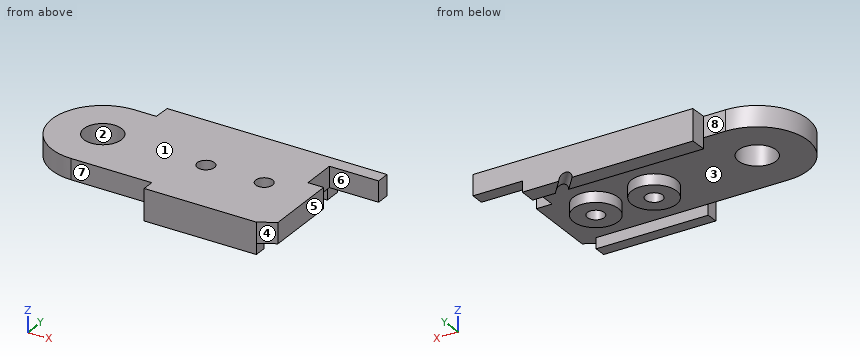
from build123d import *

# Parameters (mm, degrees)
BOSS_EXTRUDE1_DEPTH  = 2
BOSS_EXTRUDE6_DEPTH  = 2.5
CUT_EXTRUDE6_DEPTH   = 2.5
BOSS_EXTRUDE14_DEPTH = 2.3
SKETCH32_R           = 2.1
CUT_EXTRUDE7_DEPTH   = 2.3
SKETCH33_W           = 12.5
SKETCH33_H           = 1.343145751
BOSS_EXTRUDE15_DEPTH = 1.2
SKETCH35_W           = 5.479645997
SKETCH35_H           = 3.827993755
CUT_EXTRUDE8_DEPTH   = 2.4
SKETCH36_W           = 3.7
SKETCH36_H           = 1.827993755
CUT_EXTRUDE9_DEPTH   = 2.4
SKETCH37_R           = 3.9
BOSS_EXTRUDE16_DEPTH = 2.3
CUT_EXTRUDE10_DEPTH  = 5.3
SKETCH43_R           = 2.5
BOSS_EXTRUDE17_DEPTH = 1.2
SKETCH44_R           = 0.95
CUT_EXTRUDE11_DEPTH  = 9
SKETCH45_R           = 2
CUT_EXTRUDE12_DEPTH  = 2.5
SKETCH52_R           = 0.75
CUT_EXTRUDE13_DEPTH  = 10


with BuildPart() as part:
    # Sketch3 → Boss-Extrude1 (new body)
    with BuildSketch(Plane.XY):
        with BuildLine():
            Line((8, 0), (9, -2.5))
            Line((9, -2.5), (9, -7))
            Line((9, -7), (21.5, -7))
            Line((21.5, -7), (25.050252532, -4.949747468))
            ThreePointArc((25.050252532, -4.949747468), (36.467156728, -2.678784027), (30, 7))
            Line((30, 7), (27, 7.5))
            Line((27, 7.5), (5.656854249, 7.5))
            Line((5.656854249, 7.5), (5.656854249, 5.656854249))
            ThreePointArc((5.656854249, 5.656854249), (7.39103626, 3.061467459), (8, 0))
        make_face()
    extrude(amount=BOSS_EXTRUDE1_DEPTH)

    # Sketch22 → Boss-Extrude6 (add)
    with BuildSketch(Plane.XY.offset(2)):
        with BuildLine():
            Line((5.656854249, 5.656854249), (2.486790148, 5.656854249))
            Line((2.486790148, 5.656854249), (2.486790148, 7.5))
            Line((2.486790148, 7.5), (5.656854249, 7.5))
            Line((5.656854249, 7.5), (21.5, 7.5))
            Line((21.5, 7.5), (27, 7.5))
            Line((27, 7.5), (27, 2.172006245))
            Line((27, 2.172006245), (23.275126266, 2.172006245))
            Line((23.275126266, 2.172006245), (23.275126266, -5.974873734))
            Line((23.275126266, -5.974873734), (21.5, -7))
            Line((21.5, -7), (9, -7))
            Line((9, -7), (9, -2.5))
            Line((9, -2.5), (8, 0))
            ThreePointArc((8, 0), (7.39103626, 3.061467459), (5.656854249, 5.656854249))
        make_face()
    extrude(amount=BOSS_EXTRUDE6_DEPTH)

    # Sketch26 → Cut-Extrude6 (cut)
    with BuildSketch(Plane.XY.offset(2)):
        Polygon((18.098080448, 5.3), (2.530052458, 5.3), (2.530052458, 4), (18.098080448, 4), (27, 4), (27, 5.3), align=None)
    extrude(amount=CUT_EXTRUDE6_DEPTH, mode=Mode.SUBTRACT)


with BuildPart() as body_2:
    # Sketch31 → Boss-Extrude14 (new body)
    with BuildSketch(Plane.XY.offset(4.5)):
        with BuildLine():
            Line((2.432688066, 5.656854249), (0, 5.656854249))
            ThreePointArc((0, 5.656854249), (-5.656854249, 0), (0, -5.656854249))
            Line((0, -5.656854249), (9, -5.656854249))
            Line((9, -5.656854249), (9, -7))
            Line((9, -7), (21.5, -7))
            Line((21.5, -7), (23.275126266, -5.974873734))
            Line((23.275126266, -5.974873734), (23.275126266, 2.172006245))
            Line((23.275126266, 2.172006245), (27, 2.172006245))
            Line((27, 2.172006245), (27, 7.5))
            Line((27, 7.5), (2.486790148, 7.5))
            Line((2.486790148, 7.5), (2.432688066, 5.656854249))
        make_face()
    extrude(amount=BOSS_EXTRUDE14_DEPTH)

    # Sketch32 → Cut-Extrude7 (cut)
    with BuildSketch(Plane.XY.offset(6.8)):
        Circle(SKETCH32_R)
    extrude(amount=-CUT_EXTRUDE7_DEPTH, mode=Mode.SUBTRACT)

    # Sketch33 → Boss-Extrude15 (add)
    with BuildSketch(Plane.XY.offset(6.8)):
        with Locations((15.25, -6.328427125)):
            Rectangle(SKETCH33_W, SKETCH33_H)
        Polygon((2.486790148, 7.5), (21.5, 7.5), (21.5, 5.656854249), (2.432688066, 5.656854249), align=None)
    extrude(amount=BOSS_EXTRUDE15_DEPTH)


with BuildPart() as cut_extrude8_tool:
    # Sketch35 → Cut-Extrude8 (new body)
    with BuildSketch(Plane.XY.offset(6.8)):
        with Locations((24.260177002, 4.086003123)):
            Rectangle(SKETCH35_W, SKETCH35_H)
    extrude(amount=-CUT_EXTRUDE8_DEPTH)


with BuildPart() as part_1:
    add(part.part)

    # Cut-Extrude8: cut by cut_extrude8_tool
    add(cut_extrude8_tool.part, mode=Mode.SUBTRACT)

    # Sketch36 → Cut-Extrude9 (cut)
    with BuildSketch(Plane.XY.offset(4.4)):
        with Locations((25.15, 3.086003123)):
            Rectangle(SKETCH36_W, SKETCH36_H)
    extrude(amount=-CUT_EXTRUDE9_DEPTH, mode=Mode.SUBTRACT)

    # Sketch37 → Boss-Extrude16 (add)
    with BuildSketch(Plane.XY.offset(2)):
        with Locations((30, 0)):
            Circle(SKETCH37_R)
    extrude(amount=BOSS_EXTRUDE16_DEPTH)

    # Sketch39 → Cut-Extrude10 (cut, through all)
    with BuildSketch(Plane.XY.offset(4.3)):
        with BuildLine():
            Line((29, 1.732050808), (29, -1.732050808))
            ThreePointArc((29, -1.732050808), (32, 0), (29, 1.732050808))
        make_face()
    extrude(amount=-CUT_EXTRUDE10_DEPTH, mode=Mode.SUBTRACT)


with BuildPart() as body_2_1:
    add(body_2.part)

    # Cut-Extrude8: cut by cut_extrude8_tool
    add(cut_extrude8_tool.part, mode=Mode.SUBTRACT)

    # Sketch43 → Boss-Extrude17 (add)
    with BuildSketch(Plane.XY.offset(6.8)):
        with Locations((11.5, 0)):
            Circle(SKETCH43_R)
        with Locations((18, 0)):
            Circle(SKETCH43_R)
    extrude(amount=BOSS_EXTRUDE17_DEPTH)


with BuildPart() as cut_extrude11_tool:
    # Sketch44 → Cut-Extrude11 (new body, through all)
    with BuildSketch(Plane.XY.offset(8)):
        with Locations((11.5, 0)):
            Circle(SKETCH44_R)
        with Locations((18, 0)):
            Circle(SKETCH44_R)
    extrude(amount=-CUT_EXTRUDE11_DEPTH)


with BuildPart() as part_2:
    add(part_1.part)

    # Cut-Extrude11: cut by cut_extrude11_tool
    add(cut_extrude11_tool.part, mode=Mode.SUBTRACT)

    # Sketch45 → Cut-Extrude12 (cut)
    with BuildSketch(Plane(origin=(0, 0, 0), x_dir=(-1, 0, 0), z_dir=(0, 0, -1))):
        with Locations((-11.5, 0)):
            Circle(SKETCH45_R)
        with Locations((-18, 0)):
            Circle(SKETCH45_R)
    extrude(amount=-CUT_EXTRUDE12_DEPTH, mode=Mode.SUBTRACT)


with BuildPart() as body_2_2:
    add(body_2_1.part)

    # Cut-Extrude11: cut by cut_extrude11_tool
    add(cut_extrude11_tool.part, mode=Mode.SUBTRACT)

    # Sketch52 → Cut-Extrude13 (cut, along a direction that is not the sketch's normal)
    with BuildSketch(Plane.XZ.offset(-5.656854249)):
        with Locations((18.235476819, 8)):
            Circle(SKETCH52_R)
    extrude(amount=-CUT_EXTRUDE13_DEPTH, dir=(0.640410196, -0.76803306, 0), mode=Mode.SUBTRACT)


with BuildPart() as body_3:
    # Mirror1: mirrored copy
    add(body_2_2.part.mirror(Plane.XY.offset(8)))


with BuildPart() as body_4:
    # Mirror1 2: mirrored copy
    add(part_2.part.mirror(Plane.XY.offset(8)))


solid = body_3.part
Could you check a few things on this model? Use its own coordinates, in mm. Face numbers are marked on the shaded views. A direction names the side the tool comes from. Give positions to 0.01 mm unless a question says otherwise; leave off trailing zeros. Order: outer loops, then holes, each group sorted by start corner. A loop starts at its lowest first (then second) coordinate and runs counter-clockwise, first axis right, second up. Notation, with made-up numbers: (79.5, 36.5) -> (121.5, 36.5) arc R17 cw to (121.5, 45.5) -> close; hole circle Ø5 at (-1.5, 65.5). An arc over 180 degrees is marked (long way). Return JSON: item names as keys, results as strings.
1. Imagine slicing it at A-A on z = 9.95. List the corners of the cut face in (x, y) for me, then the cut area to 3 significant figures.
Answer list:
{"outline": "(0, -5.66) -> (9, -5.66) -> (9, -7) -> (21.5, -7) -> (23.28, -5.97) -> (23.28, 2.17) -> (21.52, 2.17) -> (21.52, 6) -> (27, 6) -> (27, 7.5) -> (2.49, 7.5) -> (2.43, 5.66) -> (0, 5.66) arc R5.66 ccw to start; hole circle Ø4.2 at (0, 0); hole circle Ø1.9 at (11.5, 0); hole circle Ø1.9 at (18, 0)", "area": "350 mm2"}
2. For pin 1 Ø1.5 at (y, z) = (1, 10) entering from +X; pin 2 Ø1 at (y, z) = (-6.5, 8.5) entering from +X; pin 3 Ø1.2 at (x, z) = (25.5, 10.5) entering from -Y; pin 4 Ø3 at (x, y) = (18, 0) entering from +Z, each with a flat end and sliding along its axis, tell me the tip position at first contact or that it passes through.
Answer list:
{"pin 1": "stops at x = 23.28", "pin 2": "stops at x = 21.5", "pin 3": "stops at y = 6", "pin 4": "stops at z = 11.5"}
3. Imagine slicing it at D-D on x = 22. List the corners of the cut face in (y, z) for me, then the cut area to 3 significant figures.
Answer list:
{"outline": "(-6.71, 9.2) -> (2.17, 9.2) -> (2.17, 11.5) -> (-6.71, 11.5) -> close; (6, 9.2) -> (7.5, 9.2) -> (7.5, 11.5) -> (6, 11.5) -> close", "area": "23.9 mm2"}
4. I need wall thicknesses on line 1 (Y direction, x = 11.5, z = 8.9); line 2 (Y direction, x = 11.5, z = 10.85); line 3 (Z direction, x = 1.5, y = 1.5). Which ranges of each line are inside material? Lowest first, please. Write a range as from..to.
Answer list:
{"line 1": "y = -7..-5.66, -2.5..-0.95, 0.95..2.5, 5.66..7.5", "line 2": "y = -7..-0.95, 0.95..7.5", "line 3": "z = 9.2..11.5"}
5. Imagine slicing it at B-B on x = 11.5. List the corners of the cut face in (y, z) for me.
Answer list:
{"outline": "(-7, 8) -> (-5.66, 8) -> (-5.66, 9.2) -> (-2.5, 9.2) -> (-2.5, 8) -> (-0.95, 8) -> (-0.95, 11.5) -> (-7, 11.5) -> close; (0.95, 8) -> (2.5, 8) -> (2.5, 9.2) -> (5.66, 9.2) -> (5.66, 8) -> (7.5, 8) -> (7.5, 11.5) -> (0.95, 11.5) -> close"}
6. Thinking about a two-plate mould opening in Y: for the marked faces 1, 2, 3 and 4, which applies, pulls with the +Y half, pulls with the -Y half, needs draft (parallel to the pull), parting line crosses it, or undercut?
Answer list:
{"face 1": "needs draft", "face 2": "undercut", "face 3": "undercut", "face 4": "pulls with the -Y half"}
7. On a 3-axis mill with a long thin cutter (end or side, diameter ignored), from which of +Z, -Z, +X, -X, +Y, -Y can I reach the whole of each face in a straight line? I mean the marked faces 5, 6, 7 and 8. Say none if no direction works.
Answer list:
{"face 5": "+Z, -Z, +X, -Y", "face 6": "+Z, -Z, +X", "face 7": "+Z, -Z, -X, -Y", "face 8": "+Z, -Z, -X, +Y"}
8. Imagine slicing it at C-C on y = 0. List the corners of the cut face in (x, z) for me.
Answer list:
{"outline": "(-5.66, 9.2) -> (-2.1, 9.2) -> (-2.1, 11.5) -> (-5.66, 11.5) -> close; (2.1, 9.2) -> (9, 9.2) -> (9, 8) -> (10.55, 8) -> (10.55, 11.5) -> (2.1, 11.5) -> close; (12.45, 8) -> (14, 8) -> (14, 9.2) -> (15.5, 9.2) -> (15.5, 8) -> (17.05, 8) -> (17.05, 11.5) -> (12.45, 11.5) -> close; (18.95, 8) -> (20.5, 8) -> (20.5, 9.2) -> (23.28, 9.2) -> (23.28, 11.5) -> (18.95, 11.5) -> close"}
